Source: CAD feature listing. Evaluate the final solid. Frame: model axes, mm. Face numbers are marked on the shaded views. A direction names the side the tool comes from. Give positions to 0.01 mm unless a question says otherwise; leave off trailing zeros. Order: outer loops, then holes, each group sorted by start corner. A loop starts at its lowest first (then second) coordinate and runs counter-clockwise, first axis right, second up.
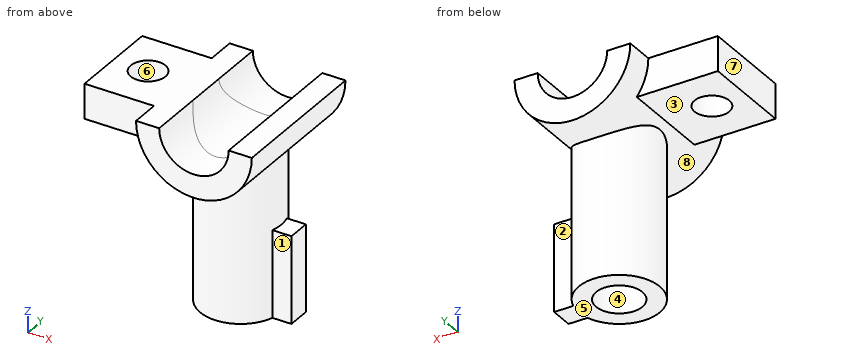
from build123d import *

# Parameters (mm, degrees)
F1_DEPTH  = 6.5
F2_W      = 8
F2_H      = 8
F3_DEPTH  = 3
F4_R      = 3.5
F5_DEPTH  = 17
F6_R      = 3
F7_DEPTH  = 9.3
F8_R      = 2
F9_DEPTH  = 12
F10_R     = 1.5
F11_DEPTH = 17.001
F13_DEPTH = 7.5


with BuildPart() as f1:
    # F0 (on Front) → F1 (new body, symmetric)
    with BuildSketch(Plane.XZ):
        with BuildLine():
            Line((-3, 0), (-5, 0))
            ThreePointArc((-5, 0), (0, -5), (5, 0))
            Line((5, 0), (3, 0))
            ThreePointArc((3, 0), (0, -3), (-3, 0))
        make_face()
    extrude(amount=F1_DEPTH, both=True)

    # F2 (on Top) → F3 (join)
    with BuildSketch(Plane.XY):
        with Locations((-7, 0)):
            Rectangle(F2_W, F2_H)
    extrude(amount=-F3_DEPTH)

    # F4 (on Top) → F5 (join)
    with BuildSketch(Plane.XY):
        Circle(F4_R)
    extrude(amount=-F5_DEPTH)

    # F6 (on Front) → F7 (cut, symmetric)
    with BuildSketch(Plane.XZ):
        Circle(F6_R)
    extrude(amount=F7_DEPTH, both=True, mode=Mode.SUBTRACT)

    # F8 (on face) → F9 (cut)
    with BuildSketch(Plane(origin=(0, 0, -17), x_dir=(1, 0, 0), z_dir=(0, 0, -1))):
        Circle(F8_R)
    extrude(amount=-F9_DEPTH, mode=Mode.SUBTRACT)

    # F10 (on face) → F11 (cut, through all)
    with BuildSketch(Plane.XY):
        with Locations((-8, 0)):
            Circle(F10_R)
    extrude(amount=-F11_DEPTH, mode=Mode.SUBTRACT)

    # F12 (on face) → F13 (join)
    with BuildSketch(Plane(origin=(0, 0, -17), x_dir=(1, 0, 0), z_dir=(0, 0, -1))):
        with BuildLine():
            ThreePointArc((3.354102, 1), (3.5, 0), (3.354102, -1))
            Line((3.354102, -1), (5, -1))
            Line((5, -1), (5, 1))
            Line((5, 1), (3.354102, 1))
        make_face()
    extrude(amount=-F13_DEPTH)


solid = f1.part
(1) Section A-A, the plane y = 0. Return loops of the section in (x, z).
(2) Pin query (flat end, axial travel): pin 1 Ø1.3 at (x, z) = (4.5, -11.5) entering from -Y; pin 2 Ø3.5 at (x, z) = (-9, -2) entering from +Y; pin 3 Ø0.5 at (x, z) = (4.5, -12) entering from +Y. Return the tip coordinate at first contact, or that it passes through.
(3) Section B-B, the plane x = -8. Return loops of the section in (y, z).
(4) Access query for the marked faces 1, 2, 3 and 4. Directions: +Z, -Z, +X, -X, +Y, -Y. A direction counts if a zero-diameter tool reaches every point of the face in a straight line with its end or side. Return the directions, or none.
(5) Line query: line 1 along X through (y, z) = (0, -10.5); line 2 along Y through (x, z) = (0, -11); line 3 along Y through (x, z) = (-8, -1.95). Output: solid intervals per line, ascending.
(6) Draft query along X for the marked faces 5, 6, 7 and 8. Return one class per face: +X half, -X half, draft (parallel to the pull), parting line (faces both ways), or undercut.
(7) Section D-D, the plane x = 0. Return loops of the section in (y, z), plus the area to 3 significant figures.
(8) Section C-C, the plane z = -14. Return loops of the section in (x, y).
Checks:
1. outline: (-11, -3) - (-9.5, -3) - (-9.5, 0) - (-11, 0) - close; (-6.5, -3) - (-4, -3) arc R5 ccw to (-3.5, -3.57) - (-3.5, -17) - (-2, -17) - (-2, -5) - (2, -5) - (2, -17) - (5, -17) - (5, -9.5) - (3.5, -9.5) - (3.5, -3.57) arc R5 ccw to (5, 0) - (3, 0) arc R3 cw to (-3, 0) - (-6.5, 0) - close
2. pin 1: stops at y = -1
2. pin 2: stops at y = 4
2. pin 3: stops at y = 1
3. outline: (-4, -3) - (-1.5, -3) - (-1.5, 0) - (-4, 0) - close; (1.5, -3) - (4, -3) - (4, 0) - (1.5, 0) - close
4. face 1: -Z, +X, -Y
4. face 2: -Z, +X, +Y
4. face 3: -Z, -X, +Y, -Y
4. face 4: -Z
5. line 1: x = -3.5 to -2, 2 to 5
5. line 2: y = -3.5 to -2, 2 to 3.5
5. line 3: y = -4 to -1.5, 1.5 to 4
6. face 5: draft
6. face 6: undercut
6. face 7: -X half
6. face 8: parting line
7. outline: (-6.5, -5) - (-3.5, -5) - (-3.5, -17) - (-2, -17) - (-2, -5) - (2, -5) - (2, -17) - (3.5, -17) - (3.5, -5) - (6.5, -5) - (6.5, -3) - (-6.5, -3) - close
7. area: 62.0 mm2
8. outline: (3.35, -1) - (5, -1) - (5, 1) - (3.35, 1) arc R3.5 ccw (long way) to start; hole circle Ø4 at (0, 0)
